CAD build for the part. Positions are in the model's coordinates, mm. A direction names the side the tool comes from. Coordinates: 2 decimals unless noted, no trailing zeros. Loops run counter-clockwise (first coordinate to the right, second up) from the corner with the lowest first, then second, coordinate; pieces in that order, holes last. Notation, with made-up numbers: (86.25, 30.5) - (143.25, 30.5) arc R20 ccw to (143.25, 34.5) - close; hole circle Ø4 at (14.5, 64.5). An arc over 180 degrees is marked (long way). Put each result on its own line as item: value.
```python
from build123d import *

# Parameters (mm, degrees)
RESSALTO_EXTRUS_O1_DEPTH = 2


with BuildPart() as part:
    # Esboço1 → Ressalto-extrusão1 (new body)
    with BuildSketch(Plane.XY):
        with BuildLine():
            Line((0, 1), (0, 26.234323652))
            ThreePointArc((0, 26.234323652), (0.216479701, 26.855689841), (0.772191883, 27.208029697))
            ThreePointArc((0.772191883, 27.208029697), (6.58904443, 27.120718638), (11.681282792, 24.30780107))
            ThreePointArc((11.681282792, 24.30780107), (11.916864982, 23.974978194), (12, 23.575780744))
            Line((12, 23.575780744), (12, 18))
            Line((12, 18), (16, 18))
            ThreePointArc((16, 18), (16.707106781, 17.707106781), (17, 17))
            Line((17, 17), (17, 7))
            ThreePointArc((17, 7), (16.707106781, 6.292893219), (16, 6))
            Line((16, 6), (13.5, 6))
            Line((13.5, 6), (12.189366094, 0.757464375))
            ThreePointArc((12.189366094, 0.757464375), (11.834635803, 0.211794562), (11.219223594, 0))
            Line((11.219223594, 0), (10, 0))
            ThreePointArc((10, 0), (9.292893219, 0.292893219), (9, 1))
            Line((9, 1), (9, 13))
            ThreePointArc((9, 13), (7, 15), (5, 13))
            Line((5, 13), (5, 1))
            ThreePointArc((5, 1), (4.707106781, 0.292893219), (4, 0))
            Line((4, 0), (1, 0))
            ThreePointArc((1, 0), (0.292893219, 0.292893219), (0, 1))
        make_face()
    extrude(amount=RESSALTO_EXTRUS_O1_DEPTH)


solid = part.part
```
Q1. Tool access for faces 1 (the flat face through (9, 7, 1)), 2 (the cylindrical face through (6.51, 27.14, 0.99)), 3 (the flat face through (12, 21, 1)): list every direction of +Z, -Z, +X, -X, +Y, -Y with a clear straight run to the whole face (end or side of a thin tool).
Determined:
face 1: +Z, -Z, -Y
face 2: +Z, -Z, +Y
face 3: +Z, -Z, +X, +Y
Q2. Slice it at D-D, the plane x = 7. Give the cut face in (y, z), then the cut area to 3 significant figures.
Determined:
outline: (15, 0) - (27, 0) - (27, 2) - (15, 2) - close
area: 24.0 mm2
Q3. Slice it at C-C, the plane y = 21.25. Give the cut face in (x, z), then the cut area to 3 significant figures.
Determined:
outline: (0, 0) - (12, 0) - (12, 2) - (0, 2) - close
area: 24.0 mm2
Q4. Mould opens along X. For faces 4 (the cylindrical face through (11.842, 0.218, 0.986)), 5 (the cylindrical face through (0.21, 26.85, 0.99)), 6 (the flat face through (5, 7, 1)), 7 (the cylindrical face through (7, 15, 1)) say: +X half, -X half, draft (parallel to the pull), parting line (faces both ways), or undercut.
Determined:
face 4: +X half
face 5: -X half
face 6: undercut
face 7: undercut
Q5. Pin check, flat tips, straight feed: pin 1 Ø2 at (x, y) = (5, 14.5) entering from -Z; pin 2 Ø0.6 at (y, z) = (19.5, 1) entering from +X; pin 3 Ø0.6 at (y, z) = (4, 0.5) entering from +X (3 decimals). Stop position of each tip, or through.
Determined:
pin 1: z = 0
pin 2: x = 12
pin 3: x = 13.075
Q6. Wall check: L1, parallel to X at y = 10.5, z = 0.6; L2, parallel to Y at x = 15.75, z = 0.6; L3, parallel to X at y = 20, z = 1. Give the ranges that are in metal, low to high. Write a range as from..to.
Determined:
L1: 0..5, 9..17
L2: 6..18
L3: 0..12
Q7. Slice it at A-A, the plane z = 1.4. Give the cut face in (x, y).
Determined:
outline: (0, 1) arc R1 ccw to (1, 0) - (4, 0) arc R1 ccw to (5, 1) - (5, 13) arc R2 cw to (9, 13) - (9, 1) arc R1 ccw to (10, 0) - (11.22, 0) arc R1 ccw to (12.19, 0.76) - (13.5, 6) - (16, 6) arc R1 ccw to (17, 7) - (17, 17) arc R1 ccw to (16, 18) - (12, 18) - (12, 23.58) arc R1 ccw to (11.68, 24.31) arc R12 ccw to (0.77, 27.21) arc R1 ccw to (0, 26.23) - close
Q8. Slice it at B-B, the plane y = 14.5. Give the cut face in (x, z).
Determined:
outline: (0, 0) - (5.68, 0) - (5.68, 2) - (0, 2) - close; (8.32, 0) - (17, 0) - (17, 2) - (8.32, 2) - close
